```python
from build123d import *

# Parameters (mm, degrees)
F0_R     = 100
F1_DEPTH = 500
F2_R     = 75
F3_DEPTH = 500.001
F4_W     = 45
F4_H     = 45
F5_DEPTH = 1890
F7_DEPTH = 500.001


with BuildPart() as f1:
    # F0 (on Top) → F1 (new body)
    with BuildSketch(Plane.XY):
        Circle(F0_R)
    extrude(amount=F1_DEPTH)

    # F2 (on face) → F3 (cut, through all)
    with BuildSketch(Plane.XY.offset(500)):
        Circle(F2_R)
    extrude(amount=-F3_DEPTH, mode=Mode.SUBTRACT)

    # F4 (on Right) → F5 (join)
    with BuildSketch(Plane.YZ):
        with Locations((0, 22.5)):
            Rectangle(F4_W, F4_H)
    extrude(amount=F5_DEPTH)

    # F6 (on face) → F7 (cut, through all)
    with BuildSketch(Plane(origin=(0, 0, 0), x_dir=(1, 0, 0), z_dir=(0, 0, -1))):
        with BuildLine():
            ThreePointArc((71.5454401063, -22.5), (74.1313294362, -11.3818274462), (75, 0))
            ThreePointArc((75, 0), (74.1313294362, 11.3818274462), (71.5454401063, 22.5))
            Line((71.5454401063, 22.5), (0, 22.5))
            Line((0, 22.5), (0, -22.5))
            Line((0, -22.5), (71.5454401063, -22.5))
        make_face()
    extrude(amount=-F7_DEPTH, mode=Mode.SUBTRACT)


solid = f1.part
```
CAD build for the part. Positions are in the model's coordinates, mm. A direction names the side the tool comes from. Round coordinates to 2 decimals unless told otherwise and drop trailing zeros. Write each loop counter-clockwise with the first axis right and the second up, starting at its lowest first coordinate (ties: lowest second). Pieces come first, ordered by that corner, then holes. Notation, with made-up numbers: (1.5, -5.5) - (42.5, -5.5) arc R22 ccw to (42.5, 4.5) - close; hole circle Ø5 at (-15, 2.5). An arc over 180 degrees is marked (long way). Return JSON: item names as keys, results as strings. Group by question number.
Item 1: Flat gauge pins, fed straight in: pin 1 Ø3 at (y, z) = (58.5, 189) entering from +X; pin 2 Ø1.5 at (y, z) = (-78.5, 390.5) entering from +X; pin 3 Ø1.5 at (x, y) = (1497.5, 15.5) entering from -Z. Where does each tip first touch, or does it go through?
Item 2: 3-axis set-ups, long thin cutter, end or side, ignore diameter. For faces 1 (the face through (71.196, 23.584, 253.5)), 2 (the face through (14, 75, 500)), 3 (the face through (981, -22.5, 22)), 4 (the face through (981, 0, 45)), 5 (the face through (981, 22.5, 22)): which of +Z, -Z, +X, -X, +Y, -Y reach the whole face in a straight line?
Item 3: Band-saw the part on A-A on x = 0. List the corners of the cut face in (y, z).
Item 4: Band-saw the part on C-C on z = 372. List the corners of the cut face in (x, y).
Item 5: Band-saw the part on B-B on y = 0. List the corners of the cut face in (x, z).
Item 6: Band-saw the part on D-D on x = 1346.5. List the corners of the cut face in (y, z).
Item 7: Probe probe 1 along Y at (x, z) = (0, 319); probe 2 along X at (y, z) = (-3, 163.5); probe 3 along Z at (x, y) = (293, 2). List the from-to ranges inside material, lowest first.
Resolved:
{
 "1": {"pin 1": "stops at x = 82.16", "pin 2": "stops at x = 62.89", "pin 3": "stops at z = 0"},
 "2": {"face 1": "+Z, -Z", "face 2": "+Z, +X, -X, +Y, -Y", "face 3": "+Z, -Z, +X, -Y", "face 4": "+Z, +X, +Y, -Y", "face 5": "+Z, -Z, +X, +Y"},
 "3": {"outline": "(-100, 0) - (-75, 0) - (-75, 500) - (-100, 500) - close; (75, 0) - (100, 0) - (100, 500) - (75, 500) - close"},
 "4": {"outline": "circle Ø200 at (0, 0); hole circle Ø150 at (0, 0)"},
 "5": {"outline": "(-100, 0) - (-75, 0) - (-75, 500) - (-100, 500) - close; (75, 0) - (1890, 0) - (1890, 45) - (100, 45) - (100, 500) - (75, 500) - close"},
 "6": {"outline": "(-22.5, 0) - (22.5, 0) - (22.5, 45) - (-22.5, 45) - close"},
 "7": {"probe 1": "y = -100 to -75, 75 to 100", "probe 2": "x = -99.95 to -74.94, 74.94 to 99.95", "probe 3": "z = 0 to 45"}
}
